Drawing for the job (mm, zero at the part's lowest x, y, z). Coordinates: 2 decimals unless noted, no trailing zeros. Write each loop counter-clockwise with the first axis right and the second up, starting at its lowest first coordinate (ties: lowest second). Pieces come first, ordered by that corner, then holes. Notation, with made-up numbers: (-34, 65.25) -> (-21, 65.25) arc R11 ccw to (-21, 72.25) -> close; hole circle Ø7 at (37.5, 59). An arc over 180 degrees is marked (long way). Answer as CSV lines item,"result".
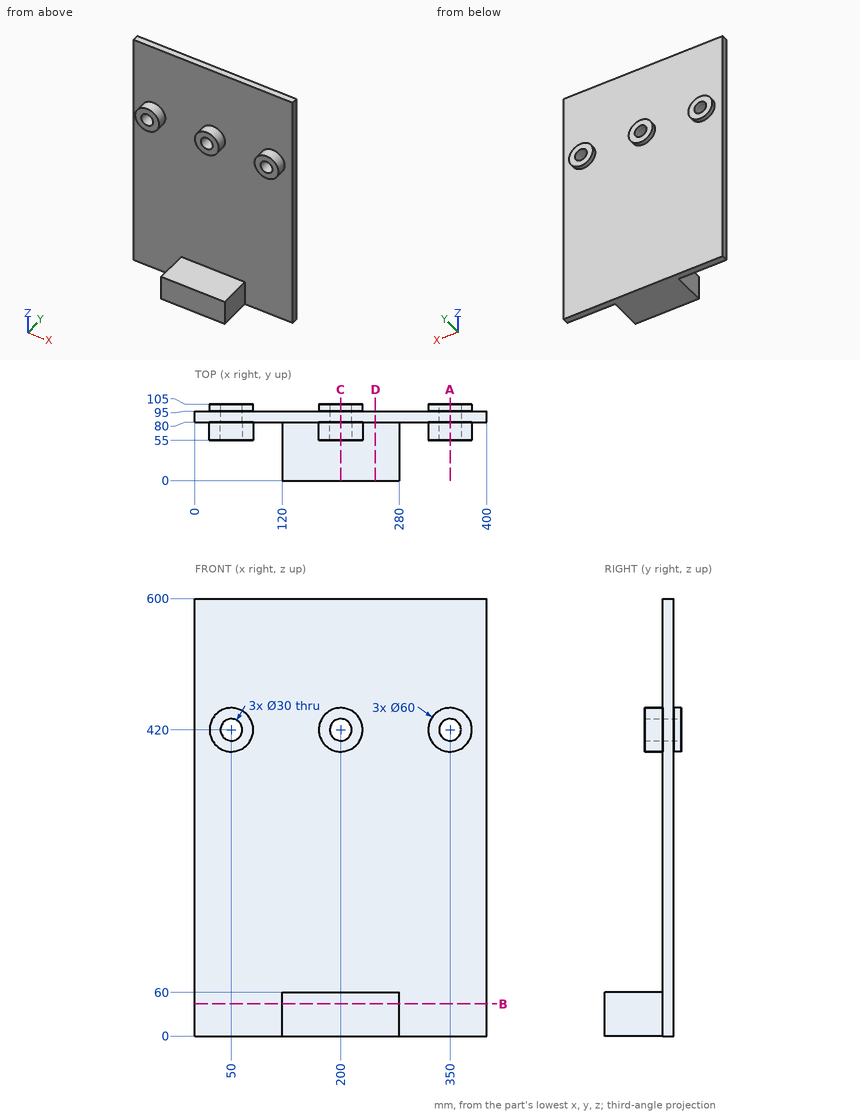
Item 1: Wall check: line 1 (Z direction, x = 200, y = 60.5); line 2 (Z direction, x = 350, y = 90); line 3 (Z direction, x = 194, y = 59). Give the ranges that are in metal, low to high. Write a range as from..to.
Answer below:
line 1,"z = 0..60, 390..405, 435..450"
line 2,"z = 0..405, 435..600"
line 3,"z = 0..60, 390.61..406.25, 433.75..449.39"
Item 2: Saw through at A-A on x = 350. Give the cut face in (y, z).
Answer below:
outline,"(55, 390) -> (80, 390) -> (80, 0) -> (95, 0) -> (95, 390) -> (105, 390) -> (105, 405) -> (55, 405) -> close; (55, 435) -> (105, 435) -> (105, 450) -> (95, 450) -> (95, 600) -> (80, 600) -> (80, 450) -> (55, 450) -> close"
Item 3: Flat gauge pins, fed straight in: pin 1 (12 mm diameter, centred on x = 225, y = 22.5, fed in from +Z); pin 2 (18 mm diameter, centred on y = 26, z = 18.5, fed in from +X); pin 3 (18 mm diameter, centred on x = 50, z = 420, fed in from +Y); pin 4 (18 mm diameter, centred on x = 53.5, z = 414.5, fed in from -Y). Where does each tip first touch, or does it go through?
Answer below:
pin 1,"stops at z = 60"
pin 2,"stops at x = 280"
pin 3,"passes through"
pin 4,"stops at y = 55"
Item 4: Saw through at B-B on z = 44. Give the cut face in (x, y), and give its area (3 significant figures).
Answer below:
outline,"(0, 80) -> (120, 80) -> (120, 0) -> (280, 0) -> (280, 80) -> (400, 80) -> (400, 95) -> (0, 95) -> close"
area,"18,800 mm2"
Item 5: Saw through at C-C on x = 200. Give the cut face in (y, z), and give its area (3 significant figures).
Answer below:
outline,"(0, 0) -> (95, 0) -> (95, 390) -> (105, 390) -> (105, 405) -> (55, 405) -> (55, 390) -> (80, 390) -> (80, 60) -> (0, 60) -> close; (55, 435) -> (105, 435) -> (105, 450) -> (95, 450) -> (95, 600) -> (80, 600) -> (80, 450) -> (55, 450) -> close"
area,"14,400 mm2"
Item 6: Saw through at D-D on x = 247.5. Give the cut face in (y, z).
Answer below:
outline,"(0, 0) -> (95, 0) -> (95, 600) -> (80, 600) -> (80, 60) -> (0, 60) -> close"
